from build123d import *

# Parameters (mm, degrees)
BOSS_EXTRUDE1_DEPTH = 4
SKETCH2_3_R         = 4.65
BOSS_EXTRUDE2_DEPTH = 8
SKETCH2_4_R         = 2.45
BOSS_EXTRUDE3_DEPTH = 15


with BuildPart() as part:
    # Sketch2 → Boss-Extrude1 (new body)
    with BuildSketch(Plane(origin=(0, 0, 0), x_dir=(1, 0, 0), z_dir=(0, 1, 0))):
        with BuildLine():
            Line((-1.1, -25), (1.1, -25))
            ThreePointArc((1.1, -25), (4.564823228, -23.564823228), (6, -20.1))
            Line((6, -20.1), (6, 20.1))
            ThreePointArc((6, 20.1), (4.564823228, 23.564823228), (1.1, 25))
            Line((1.1, 25), (-1.1, 25))
            ThreePointArc((-1.1, 25), (-4.564823228, 23.564823228), (-6, 20.1))
            Line((-6, 20.1), (-6, -20.1))
            ThreePointArc((-6, -20.1), (-4.564823228, -23.564823228), (-1.1, -25))
        make_face()
    extrude(amount=BOSS_EXTRUDE1_DEPTH)

    # Sketch2_3 → Boss-Extrude2 (add)
    with BuildSketch(Plane(origin=(0, 0, 0), x_dir=(1, 0, 0), z_dir=(0, 1, 0))):
        with Locations(Location((0, 18.75, 0), (0, 0, 270))):
            Circle(SKETCH2_3_R)
    extrude(amount=-BOSS_EXTRUDE2_DEPTH)

    # Sketch2_4 → Boss-Extrude3 (add)
    with BuildSketch(Plane(origin=(0, 0, 0), x_dir=(1, 0, 0), z_dir=(0, 1, 0))):
        with Locations(Location((0, -18.75, 0), (0, 0, 90))):
            Circle(SKETCH2_4_R)
    extrude(amount=BOSS_EXTRUDE3_DEPTH)


solid = part.part
Could you check a few things on this model? Use its own coordinates, in mm. A direction names the side the tool comes from. Give positions to 0.01 mm unless a question says otherwise; leave off trailing zeros. Order: outer loops, then holes, each group sorted by start corner. A loop starts at its lowest first (then second) coordinate and runs counter-clockwise, first axis right, second up. Notation, with made-up numbers: (-27.75, 46) - (31.25, 46) arc R17 cw to (31.25, 53) - close; hole circle Ø3 at (68, -7.75). An arc over 180 degrees is marked (long way). One line per question, with ' | ' between items. Start each with the question number.
Item 1: For faces 1 (the cylindrical face through (1.491, 9.423, 20.694)), 2 (the flat face through (6, 2, 0)), 3 (the cylindrical face through (1.397, -3.944, -14.315)), which set-ups out of +Z, -Z, +X, -X, +Y, -Y let a thin tool reach every point of the face, with its end or its side?
Item 2: I'm going to push flat-ended pins straight in: pin 1 Ø2 at (x, z) = (-3.5, -3) entering from -Y; pin 2 Ø5 at (x, y) = (0.5, -5.5) entering from +Z; pin 3 Ø3.5 at (x, z) = (-2.5, 4.5) entering from +Y. Where does each tip first touch, or does it pass through?
Item 3: I need wall thicknesses on probe 1 along Y at (x, z) = (-1.25, -8.5); probe 2 along Y at (x, z) = (0.75, 19); probe 3 along X at (y, z) = (-0.75, -18.5). Which ranges of each line are inside material? Lowest first, please. Write a range as [from, to].
Item 4: I want a section at A-A on x = 0. Write out the boundary of the cut face in (y, z).
Item 5: I want a section at C-C on y = 9.25. Write out the boundary of the cut face in (x, z).
Item 6: I want a section at D-D on z = -18.75. Write out the boundary of the cut face in (x, y).
Item 7: I want a section at B-B on z = 18.75. Write out the boundary of the cut face in (x, y), then the cut area to 3 significant figures.
Verdict:
1) face 1: +Y | face 2: +Z, -Z, +X, +Y, -Y | face 3: -Y
2) pin 1: y = 0 | pin 2: z = -14.1 | pin 3: y = 4
3) probe 1: [0, 4] | probe 2: [0, 15] | probe 3: [-4.64, 4.64]
4) outline: (-8, -23.4) - (0, -23.4) - (0, -25) - (4, -25) - (4, 16.3) - (15, 16.3) - (15, 21.2) - (4, 21.2) - (4, 25) - (0, 25) - (0, -14.1) - (-8, -14.1) - close
5) outline: circle Ø4.9 at (0, 18.75)
6) outline: (-6, 0) - (-4.65, 0) - (-4.65, -8) - (4.65, -8) - (4.65, 0) - (6, 0) - (6, 4) - (-6, 4) - close
7) outline: (-6, 0) - (6, 0) - (6, 4) - (2.45, 4) - (2.45, 15) - (-2.45, 15) - (-2.45, 4) - (-6, 4) - close | area: 102 mm^2
